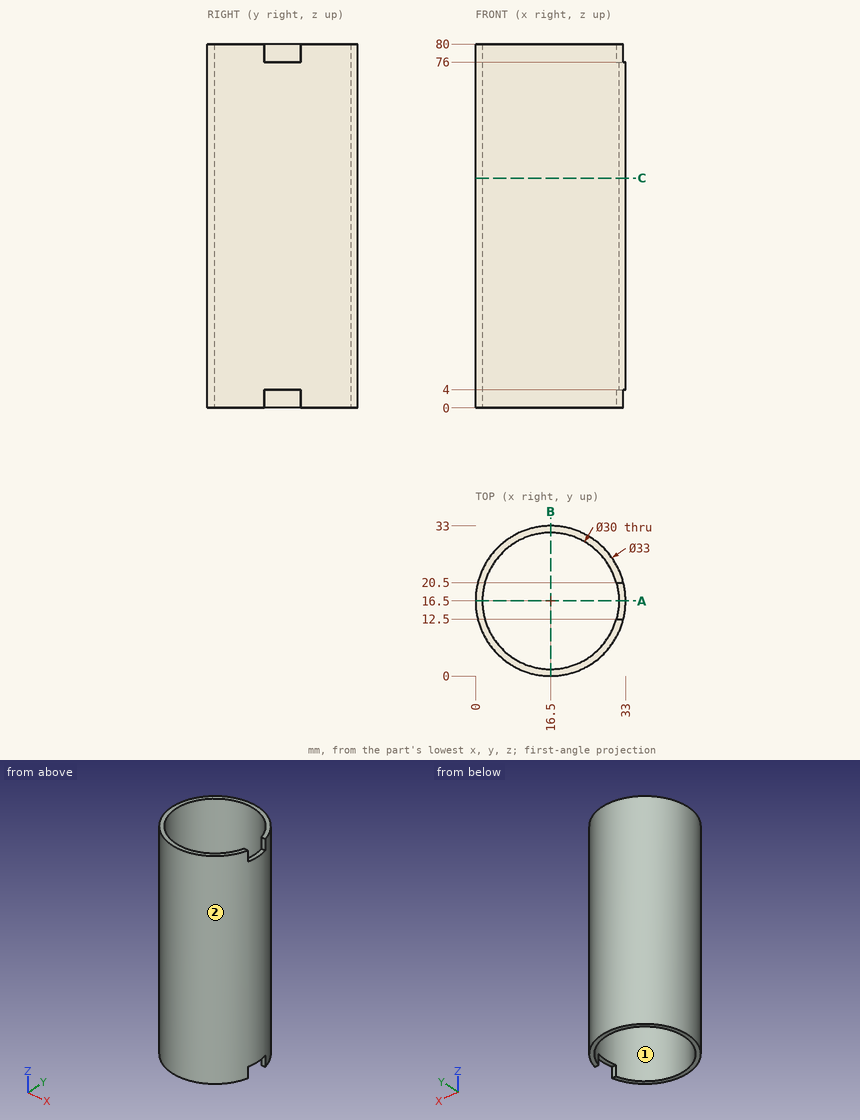
Print and shaded views of the part. All mm, measured from the part's lowest x, y and z. Give positions to 0.01 mm unless a question says otherwise; leave off trailing zeros. Loops run counter-clockwise (first coordinate to the right, second up) from the corner with the lowest first, then second, coordinate; pieces in that order, holes last. Notation, with made-up numbers: (70.5, -29.5) -> (106.5, -29.5) arc R16 cw to (106.5, -8.5) -> close; hole circle Ø9 at (1.25, 67). An arc over 180 degrees is marked (long way). Use CSV: the item, a comma, the result in double quotes. Start each with the question number.
1) Wall check: line 1 (Y direction, x = 16.5, z = 43); line 2 (X direction, y = 16, z = 38); line 3 (X direction, y = 18.5, z = 66.5). Give the ranges that are in metal, low to high.
2) Slice it at A-A on y = 16.5. Give the cut face in (x, z).
3) Slice it at B-B on x = 16.5. Give the cut face in (y, z).
4) Mould opens along Y. For the marked faces 1 and 2 say: released by +Y, released by -Y, zero draft, split by the parting line, or undercut.
5) Slice it at C-C on z = 50.5. Give the cut face in (x, y).
6) Flat gauge pins, fed straight in: pin 1 Ø0.6 at (x, y) = (32.5, 15) entering from +Z; pin 2 Ø2 at (x, y) = (28.5, 21) entering from +Z; pin 3 Ø2 at (x, y) = (31.5, 17.5) entering from -Z; pin 4 Ø1 at (x, z) = (24.5, 18.5) entering from +Y. Where does each tip first touch, or does it go through?
Computed values:
1,line 1,"y = 0 to 1.5, 31.5 to 33"
1,line 2,"x = 0.01 to 1.51, 31.49 to 32.99"
1,line 3,"x = 0.12 to 1.63, 31.37 to 32.88"
2,outline,"(0, 0) -> (1.5, 0) -> (1.5, 80) -> (0, 80) -> close; (31.5, 4) -> (33, 4) -> (33, 76) -> (31.5, 76) -> close"
3,outline,"(0, 0) -> (1.5, 0) -> (1.5, 80) -> (0, 80) -> close; (31.5, 0) -> (33, 0) -> (33, 80) -> (31.5, 80) -> close"
4,face 1,"undercut"
4,face 2,"split by the parting line"
5,outline,"circle Ø33 at (16.5, 16.5); hole circle Ø30 at (16.5, 16.5)"
6,pin 1,"stops at z = 76"
6,pin 2,"passes through"
6,pin 3,"stops at z = 4"
6,pin 4,"stops at y = 31.2"
